from build123d import *

# Parameters (mm, degrees)
SKETCH_1_R          = 1.475
EXTRUDE_1_DEPTH     = 20
SKETCH_2_R          = 1.475
SKETCH_2_R_2        = 1.375
CUT_EXTRUDE_4_DEPTH = 0.2
CUT_EXTRUDE_1_DEPTH = 7.42
FILLET_1_R          = 0.2


with BuildPart() as part:
    # 草图1 → 凸台-拉伸1 (new body)
    with BuildSketch(Plane(origin=(0, 0, 0), x_dir=(1, 0, 0), z_dir=(0, 1, 0))):
        Circle(SKETCH_1_R)
    extrude(amount=EXTRUDE_1_DEPTH)

    # 草图2 → 切除-拉伸-薄壁4 (cut)
    with BuildSketch(Plane(origin=(0, 10, 0), x_dir=(1, 0, 0), z_dir=(0, 1, 0))):
        Circle(SKETCH_2_R)
        Circle(SKETCH_2_R_2, mode=Mode.SUBTRACT)
    extrude(amount=-CUT_EXTRUDE_4_DEPTH, mode=Mode.SUBTRACT)

    # 草图3 → 切除-拉伸1 (cut)
    with BuildSketch(Plane(origin=(0, 20, 0), x_dir=(1, 0, 0), z_dir=(0, 1, 0))):
        with BuildLine():
            Line((-1.195, 0.864638653), (-1.195, -0.864638653))
            ThreePointArc((-1.195, -0.864638653), (-1.475, 0), (-1.195, 0.864638653))
        make_face()
    extrude(amount=-CUT_EXTRUDE_1_DEPTH, mode=Mode.SUBTRACT)

    # 圆角1
    fillet_1_edges = [part.edges().sort_by_distance(p)[0] for p in [
        (0.454422711, 20, 1.403255144),
    ]]
    fillet(fillet_1_edges, radius=FILLET_1_R)


solid = part.part
The listing builds one solid part. Answer for the finished solid, in the listing's coordinates (mm). A direction names the side the tool comes from. Round coordinates to 2 decimals unless told otherwise and drop trailing zeros. Loops run counter-clockwise (first coordinate to the right, second up) from the corner with the lowest first, then second, coordinate; pieces in that order, holes last. Notation, with made-up numbers: M 27,73 L 36,73 A26 cw 36,103 Z; hole C -11,27 d2. An arc over 180 degrees is marked long. Write each question's results on one line, items separated by ' | '. Start each with the question number.
1) Straight lines are drawn through the part: probe 1 along Z at (x, y) = (0.75, 11); probe 2 along Y at (x, z) = (-1.25, -0.15). For each, find the intervals that lie inside material, in ascending order.
2) Find section B-B on y = 1.5. Write down the section's boundary in (x, z) (3 decimals), plus the area to 3 significant figures.
3) Each of these flat-tipped pins is pushed along its axis until it touches: pin 1 (1.5 mm diameter, centred on x = -1, y = 7, fed in from +Z); pin 2 (1.5 mm diameter, centred on x = 0.5, z = -0.5, fed in from -Y); pin 3 (1.5 mm diameter, centred on y = 17.5, z = 1, fed in from -X) (3 decimals). Where does it stop, or does it pass through?
4) Find section C-C on y = 13.5. Write down the section's boundary in (x, z) (3 decimals), plus the area to 3 significant figures.
5) Which of the six approach directions +Z, -Z, +X, -X, +Y, -Y give full straight-line access (tool end or side, diameter ignored) to faces 1 (the flat face through (-1.195, 16, 0)), 2 (the flat face through (0, 0, 0))?
6) Find section A-A on z = 0. Write down the section's boundary in (x, y) (3 decimals).
Final values:
1) probe 1: -1.27 to 1.27 | probe 2: 0 to 12.58
2) outline: C 0,0 d2.95 | area: 6.83 mm²
3) pin 1: z = 1.45 | pin 2: y = 0 | pin 3: x = -1.195
4) outline: M -1.195,-0.865 A1.475 ccw long -1.195,0.865 Z | area: 6.51 mm²
5) face 1: +Z, -Z, -X, +Y | face 2: +Z, -Z, +X, -X, -Y
6) outline: M -1.475,0 L 1.475,0 L 1.475,9.8 L 1.375,9.8 L 1.375,10 L 1.475,10 L 1.475,19.8 A0.2 ccw 1.275,20 L -1.195,20 L -1.195,12.58 L -1.475,12.58 L -1.475,10 L -1.375,10 L -1.375,9.8 L -1.475,9.8 Z
